from build123d import *

# Parameters (mm, degrees)
F0_R     = 1.375
F0_R_2   = 1.25
F0_R_3   = 8
F0_R_4   = 9.5
F0_R_5   = 3
F1_DEPTH = 4
F2_R     = 3


with BuildPart() as f1:
    # F0 (on Top) → F1 (new body)
    with BuildSketch(Plane.XY):
        with BuildLine():
            Line((-4.7679491924, -48.5), (79.5, -48.5))
            Line((79.5, -48.5), (79.5, 48.5))
            Line((79.5, 48.5), (-79.5, 48.5))
            Line((-79.5, 48.5), (-79.5, -48.5))
            Line((-79.5, -48.5), (-64.2320508076, -48.5))
            ThreePointArc((-64.2320508076, -48.5), (-62.5, -47.5), (-60.7679491924, -48.5))
            Line((-60.7679491924, -48.5), (-8.2320508076, -48.5))
            ThreePointArc((-8.2320508076, -48.5), (-6.5, -47.5), (-4.7679491924, -48.5))
        make_face()
        with Locations((-59, -21.75)):
            Circle(F0_R, mode=Mode.SUBTRACT)
        with Locations((-10, -21.75)):
            Circle(F0_R, mode=Mode.SUBTRACT)
        with Locations((-72.275, 33.5)):
            Circle(F0_R_2, mode=Mode.SUBTRACT)
        with Locations((-59, 36.25)):
            Circle(F0_R, mode=Mode.SUBTRACT)
        with Locations((-10, 36.25)):
            Circle(F0_R, mode=Mode.SUBTRACT)
        with Locations((39.5, -9.5)):
            Circle(F0_R_3, mode=Mode.SUBTRACT)
        with Locations((21.5, 13.5)):
            Circle(F0_R_4, mode=Mode.SUBTRACT)
        with Locations((49.5, 18.5)):
            Circle(F0_R_5, mode=Mode.SUBTRACT)
        with Locations((72.275, 33.5)):
            Circle(F0_R_2, mode=Mode.SUBTRACT)
        with BuildLine():
            Line((-8.2320508076, -48.5), (-4.7679491924, -48.5))
            ThreePointArc((-4.7679491924, -48.5), (-6.5, -47.5), (-8.2320508076, -48.5))
        make_face()
        with BuildLine():
            Line((-64.2320508076, -48.5), (-60.7679491924, -48.5))
            ThreePointArc((-60.7679491924, -48.5), (-62.5, -47.5), (-64.2320508076, -48.5))
        make_face()
    extrude(amount=F1_DEPTH)

    # F2
    f2_edges = [f1.edges().sort_by_distance(p)[0] for p in [
        (-79.5, 48.5, 2),
        (79.5, 48.5, 2),
        (79.5, -48.5, 2),
        (-79.5, -48.5, 2),
    ]]
    fillet(f2_edges, radius=F2_R)


solid = f1.part
Design review of the part built by this model. Coordinates are the model's own, in mm. Round coordinates to 2 decimals unless told otherwise and drop trailing zeros. Order: outer loops, then holes, each group sorted by start corner. A loop starts at its lowest first (then second) coordinate and runs counter-clockwise, first axis right, second up.
1) For L1, parallel to Y at x = 21.5, z = 1.15; L2, parallel to X at y = -9, z = 1.45; L3, parallel to X at y = 35.5, z = 3.8, list the stretches that pass through material, from the lowest coordinate up.
The answers:
L1: y = -48.5 to 4, 23 to 48.5
L2: x = -79.5 to 31.52, 47.48 to 79.5
L3: x = -79.5 to -60.15, -57.85 to -11.15, -8.85 to 79.5
2) Consider section A-A (x = 49.5). State the section outline as (y, z) points, plus the area to 3 significant figures.
The answers:
outline: (-48.5, 0) - (15.5, 0) - (15.5, 4) - (-48.5, 4) - close; (21.5, 0) - (48.5, 0) - (48.5, 4) - (21.5, 4) - close
area: 364 mm2
3) Consider section B-B (y = 8). State the section outline as (x, z) points, plus the area to 3 significant figures.
The answers:
outline: (-79.5, 0) - (13.75, 0) - (13.75, 4) - (-79.5, 4) - close; (29.25, 0) - (79.5, 0) - (79.5, 4) - (29.25, 4) - close
area: 574 mm2
4) Consider section C-C (z = 3.4). Count the separate pieces of the cut face and the enclosed holes in it, plus the area to 3 significant figures.
The answers:
separate pieces: 1
enclosed holes: 9
area: 14,900 mm2
5) Clearance check with flat-ended pins moving along their axes: pin 1 Ø9.5 at (x, y) = (49.5, 18.5) entering from -Z; pin 2 Ø2.5 at (x, y) = (-59, 36.25) entering from -Z. State where each tip first meets the part, or that it passes through.
The answers:
pin 1: stops at z = 0
pin 2: passes through
6) Consider section D-D (y = 18.5). State the section outline as (x, z) points, plus the area to 3 significant figures.
The answers:
outline: (-79.5, 0) - (13.42, 0) - (13.42, 4) - (-79.5, 4) - close; (29.58, 0) - (46.5, 0) - (46.5, 4) - (29.58, 4) - close; (52.5, 0) - (79.5, 0) - (79.5, 4) - (52.5, 4) - close
area: 547 mm2
7) Draft analysis for pull direction X (two halves, no side actions). For faces 1 (the flat face through (-1, 1, 4)), 2 (the flat face through (79.5, -1, 2)), 3 (the cylindrical face through (-78.64, -47.6, 2.03)), 4 (the cylindrical face through (33.151, -14.368, 1.972)), state which applies: released by +X, released by -X, zero draft, split by the parting line, or undercut.
The answers:
face 1: zero draft
face 2: released by +X
face 3: released by -X
face 4: undercut
